from build123d import *

# Parameters (mm, degrees)
F0_R     = 14.946104
F0_R_2   = 15.580655
F1_DEPTH = 38.354
F2_R     = 9.594843
F3_DEPTH = 67.818
F5_DEPTH = 58.928


with BuildPart() as f1:
    # F0 (on Top) → F1 (new body)
    with BuildSketch(Plane.XY):
        with BuildLine():
            ThreePointArc((152.780443, -67.56109), (220.341533, 0), (152.780443, 67.56109))
            Line((152.780443, 67.56109), (-152.780443, 67.56109))
            ThreePointArc((-152.780443, 67.56109), (-220.341533, 0), (-152.780443, -67.56109))
            Line((-152.780443, -67.56109), (152.780443, -67.56109))
        make_face()
        with Locations((-152.780443, 0)):
            Circle(F0_R, mode=Mode.SUBTRACT)
        with Locations((152.780443, 0)):
            Circle(F0_R_2, mode=Mode.SUBTRACT)
    extrude(amount=F1_DEPTH)

    # F2 (on Right) → F3 (join, symmetric)
    with BuildSketch(Plane.YZ):
        with BuildLine():
            ThreePointArc((31.568192, 97.693309), (0, 129.261501), (-31.568192, 97.693309))
            Line((-31.568192, 97.693309), (-31.568192, 38.354))
            Line((-31.568192, 38.354), (31.568192, 38.354))
            Line((31.568192, 38.354), (31.568192, 97.693309))
        make_face()
        with Locations((0, 97.693309)):
            Circle(F2_R, mode=Mode.SUBTRACT)
    extrude(amount=F3_DEPTH, both=True)

    # F4 (on Front) → F5 (cut, symmetric)
    with BuildSketch(Plane.XZ):
        with BuildLine():
            Line((26.493635, 63.081741), (26.493635, 133.099258))
            Line((26.493635, 133.099258), (-26.493635, 133.099258))
            Line((-26.493635, 133.099258), (-26.493635, 63.081741))
            ThreePointArc((-26.493635, 63.081741), (0, 48.626888), (26.493635, 63.081741))
        make_face()
    extrude(amount=F5_DEPTH, both=True, mode=Mode.SUBTRACT)


solid = f1.part
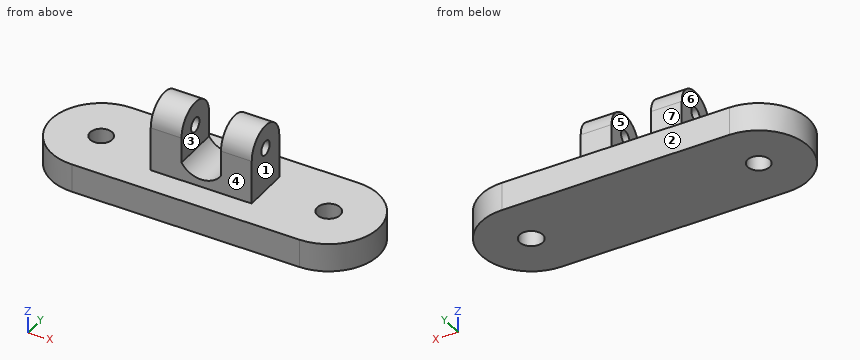
Verification items for the finished model (mm, model axes). Face numbers are marked on the shaded views. A direction names the side the tool comes from. Coordinates: 2 decimals unless noted, no trailing zeros. Write each loop counter-clockwise with the first axis right and the second up, starting at its lowest first coordinate (ties: lowest second). Pieces come first, ordered by that corner, then holes. Notation, with made-up numbers: M 28,5 L 76,5 A36 cw 76,39 Z; hole C -30,58 d5. An arc over 180 degrees is marked long. Use a Markdown table: item, result.
Q1. Sectioned sample at B-B, the plane y = 0. Record the boundary of the cut face in (x, z).
Reply:
| item | result |
|---|---|
| outline | M -220.34,0 L -167.73,0 L -167.73,38.35 L -220.34,38.35 Z; M -137.83,0 L 137.2,0 L 137.2,38.35 L 67.82,38.35 L 67.82,88.1 L 26.49,88.1 L 26.49,63.08 A31.51 cw -26.49,63.08 L -26.49,88.1 L -67.82,88.1 L -67.82,38.35 L -137.83,38.35 Z; M -67.82,107.29 L -26.49,107.29 L -26.49,129.26 L -67.82,129.26 Z; M 26.49,107.29 L 67.82,107.29 L 67.82,129.26 L 26.49,129.26 Z; M 168.36,0 L 220.34,0 L 220.34,38.35 L 168.36,38.35 Z |
Q2. Thickness scan on line 1 (X direction, y = -22, z = 111.5); line 2 (Y direction, x = -38, z = 39.5); line 3 (Z direction, x = 183, y = 19). Record the ranges inside material, lowest first.
Reply:
| item | result |
|---|---|
| line 1 | x = -67.82 to -26.49, 26.49 to 67.82 |
| line 2 | y = -31.57 to 31.57 |
| line 3 | z = 0 to 38.35 |
Q3. Sectioned sample at A-A, the plane z = 74. Record the boundary of the cut face in (x, y).
Reply:
| item | result |
|---|---|
| outline | M -67.82,-31.57 L -26.49,-31.57 L -26.49,31.57 L -67.82,31.57 Z; M 26.49,-31.57 L 67.82,-31.57 L 67.82,31.57 L 26.49,31.57 Z |
Q4. Sectioned sample at C-C, the plane x = 141.5. Record the boundary of the cut face in (y, z), plus the area to 3 significant figures.
Reply:
| item | result |
|---|---|
| outline | M -67.56,0 L -10.75,0 L -10.75,38.35 L -67.56,38.35 Z; M 10.75,0 L 67.56,0 L 67.56,38.35 L 10.75,38.35 Z |
| area | 4,360 mm² |
Q5. Go/stop test with flat-tipped pins: P1, Ø3, axis at x = 111.5, y = 51.5, coming from the +Z side; P2, Ø6, axis at x = 68, z = 83, coming from the +Y side; P3, Ø18, axis at x = 33, z = 81, coming from the -Y side. Record where each tip stops, or that it passes through.
Reply:
| item | result |
|---|---|
| P1 | stops at z = 38.35 |
| P2 | stops at y = 31.57 |
| P3 | stops at y = -31.57 |
Q6. Set-up check for the marked faces 4, 5, 6 and 7: record each of +Z, -Z, +X, -X, +Y, -Y from which the full face is reachable in a straight line by a thin tool's end or side.
Reply:
| item | result |
|---|---|
| face 4 | +Z, +X, -X, -Y |
| face 5 | +Z, +Y, -Y |
| face 6 | +Z, -X, +Y, -Y |
| face 7 | +Z, +X, -X, +Y |
Q7. Sectioned sample at D-D, the plane z = 32. Record the boundary of the cut face in (x, y), plus the area to 3 significant figures.
Reply:
| item | result |
|---|---|
| outline | M -152.78,-67.56 L 152.78,-67.56 A67.56 ccw 152.78,67.56 L -152.78,67.56 A67.56 ccw Z; hole C -152.78,0 d29.89; hole C 152.78,0 d31.16 |
| area | 54,200 mm² |
Q8. Draft check along X on the marked faces 1, 2 and 3. Enter one of: +X half, -X half, draft (parallel to the pull), parting line (faces both ways), or undercut.
Reply:
| item | result |
|---|---|
| face 1 | +X half |
| face 2 | draft |
| face 3 | undercut |
